Source: CAD feature listing. Evaluate the final solid. Frame: model axes, mm. Face numbers are marked on the shaded views. A direction names the side the tool comes from. Coordinates: 2 decimals unless noted, no trailing zeros. Order: outer loops, then holes, each group sorted by start corner. A loop starts at its lowest first (then second) coordinate and runs counter-clockwise, first axis right, second up.
Item 1: Ray query, line 1 (Z direction, x = 8.5, y = 1.3) (3 decimals); line 2 (X direction, y = 2.5, z = -8); line 3 (Z direction, x = 8.5, y = 2.55) (3 decimals). Return the intervals inside material, ascending.
Item 2: Mould query, pull axis X, two halves, no side actions, for the marked faces 1, 2 and 3. Classes: released by +X, released by -X, zero draft, split by the parting line, or undercut.
Item 3: Section C-C on y = -1.5. Return the cut outline in (x, z) (3 decimals), then the cut area to 3 significant figures.
Item 4: Section D-D on z = 8. Return the cut outline in (x, y), then the cut area to 3 significant figures.
Item 5: Reachability of the marked faces 4, 5, 6 and 7 from +Z, -Z, +X, -X, +Y, -Y: full face, straight path, thin tool, end or side. Return the list, or none.
Item 6: Section A-A on x = 10. Return the cut outline in (y, z) (3 decimals), then the cut area to 3 significant figures.
Item 7: Contact query for flat-ended pins moving along their axis: P1, Ø2.5, axis at x = -8.5, z = 0.875, coming from the +Y side; P2, Ø4, axis at x = 8.5, z = 7.5, coming from the +Y side; P3, Ø5, axis at x = 3, y = 6.5, coming from the -Z side; P4, Ø5, axis at x = 3.5, z = 6.5, coming from the +Y side. Output: stop coordinate, or through.
Item 8: Section B-B on z = -0.5. Return the cut outline in (x, y), then the cut area to 3 significant figures.
from build123d import *

# Parameters (mm, degrees)
DODANIE_WYCI_GNI_CIE1_DEPTH = 12
SZKIC3_R                    = 2
WYTNIJ_WYCI_GNI_CIE1_DEPTH  = 12
SZKIC5_R                    = 4
WYTNIJ_WYCI_GNI_CIE4_DEPTH  = 10
SZKIC12_R                   = 2.5
WYTNIJ_WYCI_GNI_CIE8_DEPTH  = 11.0000001
SZKIC13_R                   = 2
WYTNIJ_WYCI_GNI_CIE9_DEPTH  = 25.5000001


with BuildPart() as part:
    # Szkic1 → Obrót1 (revolve)
    with BuildSketch(Plane(origin=(0, 0, 0), x_dir=(1, 0, 0), z_dir=(0, 1, 0))):
        Polygon((2.5, -0.875), (2.5, 9.125), (-2.5, 9.125), (-2.5, 4.125), (-12.5, 4.125), (-12.5, -0.875), align=None)
    revolve(axis=Axis((-12.5, 0, 0.875), (1, 0, 0)))

    # Szkic2 → Dodanie-wyciągnięcie1 (add)
    with BuildSketch(Plane(origin=(2.5, 0, 0), x_dir=(0, 0, -1), z_dir=(1, 0, 0))):
        with BuildLine():
            Line((-10.875, 0), (9.125, 0))
            ThreePointArc((9.125, 0), (-0.875, 10), (-10.875, 0))
        make_face()
    extrude(amount=DODANIE_WYCI_GNI_CIE1_DEPTH)

    # Szkic3 → Wytnij-wyciągnięcie1 (cut)
    with BuildSketch(Plane(origin=(0, 0, 0), x_dir=(-1, 0, 0), z_dir=(0, -1, 0))):
        with Locations((-8.5, -5.625)):
            Circle(SZKIC3_R)
        with Locations((-8.5, 3.875)):
            Circle(SZKIC3_R)
    extrude(amount=-WYTNIJ_WYCI_GNI_CIE1_DEPTH, mode=Mode.SUBTRACT)

    # Szkic5 → Wytnij-wyciągnięcie4 (cut)
    with BuildSketch(Plane(origin=(0, 4.5, 0), x_dir=(-1, 0, 0), z_dir=(0, -1, 0))):
        with Locations((-8.5, -5.625)):
            Circle(SZKIC5_R)
    extrude(amount=-WYTNIJ_WYCI_GNI_CIE4_DEPTH, mode=Mode.SUBTRACT)

    # Szkic12 → Wytnij-wyciągnięcie8 (cut, through all)
    with BuildSketch(Plane(origin=(0, 0, 0), x_dir=(1, 0, 0), z_dir=(0, 1, 0))):
        with Locations((14.5, -0.88)):
            Circle(SZKIC12_R)
    extrude(amount=WYTNIJ_WYCI_GNI_CIE8_DEPTH, mode=Mode.SUBTRACT)

    # Szkic13 → Wytnij-wyciągnięcie9 (cut, through all)
    with BuildSketch(Plane(origin=(0, 14.5, 0), x_dir=(1, 0, 0), z_dir=(0, 1, 0))):
        with Locations((-8.5, -0.875)):
            Circle(SZKIC13_R)
    extrude(amount=-WYTNIJ_WYCI_GNI_CIE9_DEPTH, mode=Mode.SUBTRACT)


solid = part.part
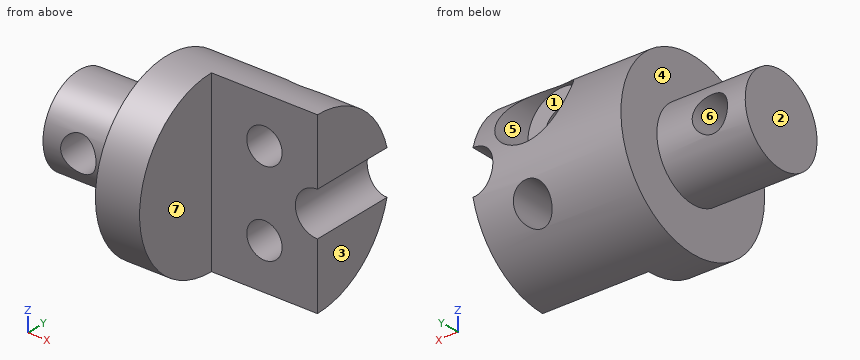
Answer list:
1. line 1: z = -9.04 to -5.875, -1.875 to 3.625, 7.625 to 10.79
1. line 2: x = -2.5 to 14.5
1. line 3: z = -8.794 to -5.875, -1.875 to 3.625, 7.625 to 10.544
2. face 1: undercut
2. face 2: released by -X
2. face 3: released by +X
3. outline: (-12.5, -3.895) - (-2.5, -3.895) - (-2.5, -9.012) - (2.5, -9.012) - (2.5, 10.762) - (-2.5, 10.762) - (-2.5, 5.645) - (-12.5, 5.645) - close; hole circle Ø4 at (-8.5, 0.875)
3. area: 182 mm2
4. outline: (-2.5, -7.02) - (2.5, -7.02) - (2.5, 0) - (14.5, 0) - (14.5, 7.02) - (11.72, 7.02) - (11.72, 4.5) - (5.28, 4.5) - (5.28, 7.02) - (-2.5, 7.02) - close
4. area: 138 mm2
5. face 4: -X
5. face 5: +Y
5. face 6: +Y, -Y
5. face 7: +Z, -Z, +X, -Y
6. outline: (0, -9.125) arc R10 ccw to (7.945, -5.198) - (0, -5.198) - close; (0, -2.552) - (9.394, -2.552) arc R10 ccw to (9.946, 1.917) - (4.5, 1.917) - (4.5, 4.302) - (0, 4.302) - close; (0, 6.948) - (4.5, 6.948) - (4.5, 9.333) - (5.335, 9.333) arc R10 ccw to (0, 10.875) - close
6. area: 92.8 mm2
7. P1: passes through
7. P2: stops at y = 4.5
7. P3: stops at z = -8.29
7. P4: stops at y = 9.5
8. outline: (-12.5, -4.81) - (-9.95, -4.81) - (-9.95, 4.81) - (-12.5, 4.81) - close; (-7.05, -4.81) - (-2.5, -4.81) - (-2.5, -9.91) - (2.5, -9.91) - (2.5, 0) - (12.42, 0) - (12.42, 9.91) - (-2.5, 9.91) - (-2.5, 4.81) - (-7.05, 4.81) - close
8. area: 265 mm2
